For this review, use the dimensioned drawing (mm, ordinates from the lowest corner) and the shaded views. A direction names the side the tool comes from. Round coordinates to 2 decimals unless told otherwise and drop trailing zeros. Loops run counter-clockwise (first coordinate to the right, second up) from the corner with the lowest first, then second, coordinate; pieces in that order, holes last. Notation, with made-up numbers: M -36.5,18 L -25.5,18 A9 ccw -25.5,30 Z; hole C -2,0.5 d1. An arc over 180 degrees is marked long. Use a Markdown table: item, result. Add a question column.
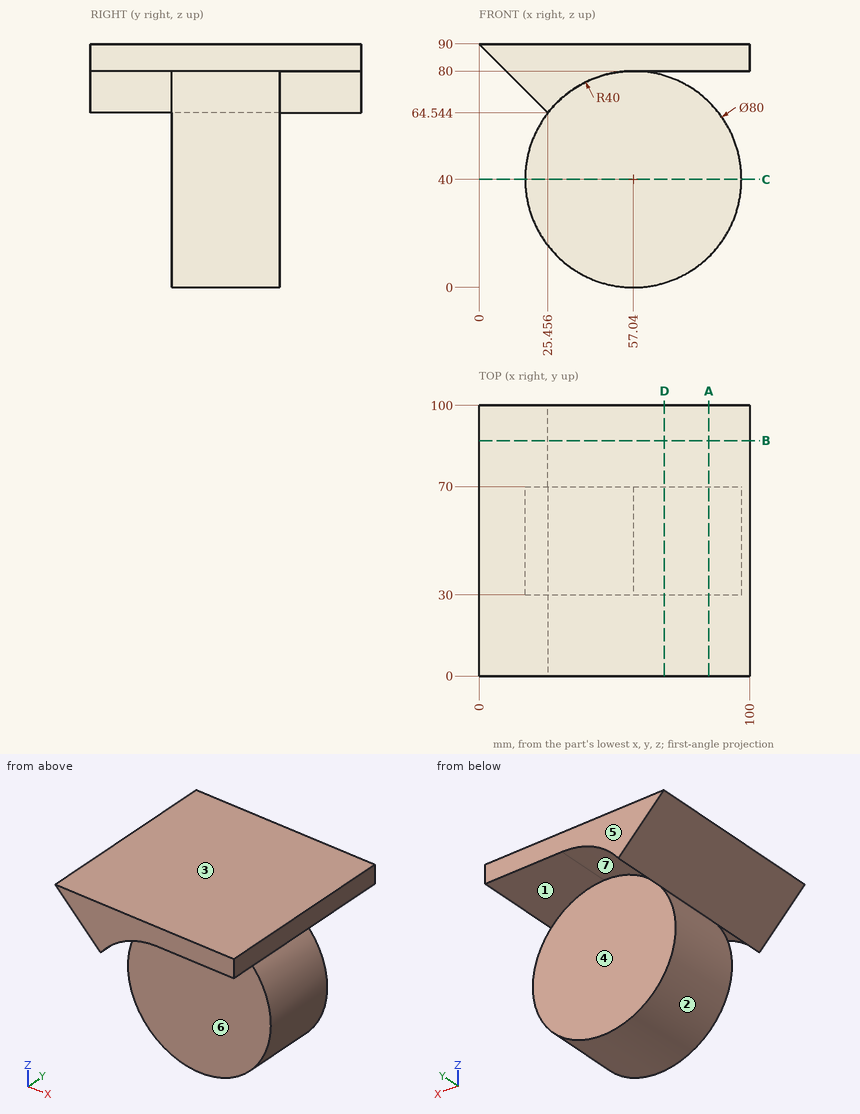
(1) Consider section B-B, the plane y = 87. Give the boundary of the cut face in (x, z), then the cut area to 3 significant figures.
(2) Consider section D-D, the plane x = 68.5. Give the boundary of the cut face in (y, z), then the cut area to 3 significant figures.
(3) To check wall thickness, follow probe 1 along X at (y, z) = (35, 40); probe 2 along Y at (x, z) = (24, 51.5); probe 3 along Z at (x, y) = (67, 14.5). State the ranges of each line that lie inside material, in increasing order.
(4) Draft analysis for pull direction Z (two halves, no side actions). For the marked faces 1, 2, 3 and 4, state which applies: released by +Z, released by -Z, zero draft, split by the parting line, or undercut.
(5) Insertion check: pin 1 Ø1 at (y, z) = (36.5, 20.5) entering from +X; pin 2 Ø24 at (x, z) = (67.5, 30) entering from +Y; pin 3 Ø8 at (x, y) = (64, 73.5) entering from -Z; pin 4 Ø3 at (x, z) = (16.5, 25.5) entering from -Y. Each pin has a flat end and moves straight along its axis. Give the tip position at first contact, or say it passes through.
(6) For the marked faces 5, 6 and 7, list the 3-axis set-ups (+Z, -Z, +X, -X, +Y, -Y) from which the entire face can be reached by the end or side of a thin tool; tool diameter is ignored.
(7) Consider section A-A, the plane x = 85. Give the boundary of the cut face in (y, z) (1 decimal).
(8) Consider section C-C, the plane z = 40. Give the boundary of the cut face in (x, y), then the cut area to 3 significant figures.
Found:
| question | item | result |
|---|---|---|
| 1 | outline | M 0,90 L 25.46,64.54 A40 cw 57.04,80 L 100,80 L 100,90 Z |
| 1 | area | 1,220 mm^2 |
| 2 | outline | M 0,80 L 100,80 L 100,90 L 0,90 Z; M 30,1.68 L 70,1.68 L 70,78.32 L 30,78.32 Z |
| 2 | area | 4,070 mm^2 |
| 3 | probe 1 | x = 17.04 to 97.04 |
| 3 | probe 2 | y = 30 to 70 |
| 3 | probe 3 | z = 80 to 90 |
| 4 | face 1 | undercut |
| 4 | face 2 | undercut |
| 4 | face 3 | released by +Z |
| 4 | face 4 | zero draft |
| 5 | pin 1 | stops at x = 92.24 |
| 5 | pin 2 | stops at y = 70 |
| 5 | pin 3 | stops at z = 0.32 |
| 5 | pin 4 | passes through |
| 6 | face 5 | +Z, -Z, +X, -X, +Y |
| 6 | face 6 | -Z, +X, -Y |
| 6 | face 7 | -Z, +X, +Y |
| 7 | outline | M 0,80 L 100,80 L 100,90 L 0,90 Z; M 30,11.4 L 70,11.4 L 70,68.6 L 30,68.6 Z |
| 8 | outline | M 17.04,30 L 97.04,30 L 97.04,70 L 17.04,70 Z |
| 8 | area | 3,200 mm^2 |
